from build123d import *

# Parameters (mm, degrees)
SKETCH_1_W      = 42
SKETCH_1_H      = 149
EXTRUDE_1_DEPTH = 3
SKETCH_2_W      = 25
SKETCH_2_H      = 12.5
EXTRUDE_2_DEPTH = 3
FILLET_1_R      = 1
SKETCH_3_W      = 6
SKETCH_3_H      = 4
EXTRUDE_3_DEPTH = 3
FILLET_2_R      = 2


with BuildPart() as part:
    # 草图1 → 凸台-拉伸1 (new body)
    with BuildSketch(Plane.XY):
        Rectangle(SKETCH_1_W, SKETCH_1_H)
    extrude(amount=EXTRUDE_1_DEPTH)

    # 草图2 → 凸台-拉伸2 (add)
    with BuildSketch(Plane.XY.offset(3)):
        with Locations((33.5, -68.25)):
            Rectangle(SKETCH_2_W, SKETCH_2_H)
        with Locations((-33.5, -68.25)):
            Rectangle(SKETCH_2_W, SKETCH_2_H)
        with Locations((-33.5, 68.25)):
            Rectangle(SKETCH_2_W, SKETCH_2_H)
        with Locations((33.5, 68.25)):
            Rectangle(SKETCH_2_W, SKETCH_2_H)
    extrude(amount=-EXTRUDE_2_DEPTH)

    # 圆角1
    fillet_1_edges = [part.edges().sort_by_distance(p)[0] for p in [
        (46, -74.5, 1.5),
        (46, -62, 1.5),
        (-46, -62, 1.5),
        (-46, -74.5, 1.5),
        (-46, 74.5, 1.5),
        (-46, 62, 1.5),
        (46, 62, 1.5),
        (46, 74.5, 1.5),
    ]]
    fillet(fillet_1_edges, radius=FILLET_1_R)

    # 草图3 → 凸台-拉伸3 (add)
    with BuildSketch(Plane(origin=(0, 0, 0), x_dir=(-1, 0, 0), z_dir=(0, 0, -1))):
        with Locations((38.15, 60)):
            Rectangle(SKETCH_3_W, SKETCH_3_H)
        with Locations((-38.15, 60)):
            Rectangle(SKETCH_3_W, SKETCH_3_H)
        with Locations((-38.15, -60)):
            Rectangle(SKETCH_3_W, SKETCH_3_H)
        with Locations((38.15, -60)):
            Rectangle(SKETCH_3_W, SKETCH_3_H)
    extrude(amount=-EXTRUDE_3_DEPTH)

    # 圆角2
    fillet_2_edges = [part.edges().sort_by_distance(p)[0] for p in [
        (-41.15, -58, 1.5),
        (-35.15, -58, 1.5),
        (-35.15, -62, 1.5),
        (41.15, -58, 1.5),
        (35.15, -62, 1.5),
        (35.15, -58, 1.5),
        (35.15, 58, 1.5),
        (41.15, 58, 1.5),
        (-35.15, 58, 1.5),
        (-35.15, 62, 1.5),
        (-41.15, 58, 1.5),
        (41.15, 62, 1.5),
    ]]
    fillet(fillet_2_edges, radius=FILLET_2_R - 0.0001)  # a hair under: the kernel refuses the full size


solid = part.part
Verification items for the finished model (mm, model axes). A direction names the side the tool comes from. Coordinates: 2 decimals unless noted, no trailing zeros. Order: outer loops, then holes, each group sorted by start corner. A loop starts at its lowest first (then second) coordinate and runs counter-clockwise, first axis right, second up. Notation, with made-up numbers: M 33,-39 L 46,-39 A24 cw 46,-8 Z; hole C 14,46.5 d3. An arc over 180 degrees is marked long. One line per item, written item: value. Start each with the question number.
Item 1: Depth check by flat-ended pin: P1, Ø1.5, axis at y = -12.5, z = 1.5, coming from the -X side; P2, Ø1, axis at y = -61, z = 1.5, coming from the -X side; P3, Ø0.6, axis at y = -61, z = 1, coming from the +X side. Enter the tip coordinate at first touch or a pass-through.
Item 2: Mould release check, pull along Y, two halves, no side actions. Record for faces 1 (the flat face through (-1, -74.5, 2)), 2 (the flat face through (21, -1, 1)), 3 (the flat face through (-46, 68, 2)): pulls with the +Y half, pulls with the -Y half, needs draft (parallel to the pull), parting line crosses it, or undercut.
Item 3: Thickness scan on probe 1 along Y at (x, z) = (27, 1.8); probe 2 along X at (y, z) = (23, 1.4); probe 3 along X at (y, z) = (59.5, 1.35). Record the ranges inside material, lowest first.
Item 4: Access from +Z, -Z, +X, -X, +Y, -Y to the whole of each face (thin tool, end or side, straight path). Record for faces 4 (the flat face through (-1, 1, 0)), 5 (the flat face through (28, 62, 2)), 6 (the flat face through (43, -62, 2)), 7 (the flat face through (-43, -62, 2)), 8 (the flat face through (-46, -68, 2)).
Item 5: Sectioned sample at A-A on y = -11.5. Record the cut outline in (x, z).
Calculated:
1. P1: x = -21
1. P2: x = -41.15
1. P3: x = 41.15
2. face 1: pulls with the -Y half
2. face 2: undercut
2. face 3: needs draft
3. probe 1: -74.5 to -62, 62 to 74.5
3. probe 2: -21 to 21
3. probe 3: -41.09 to -35.21, -21 to 21, 35.21 to 41.09
4. face 4: -Z, +X, -X, +Y, -Y
4. face 5: +Z, -Z
4. face 6: +Z, -Z, +X
4. face 7: +Z, -Z, -X
4. face 8: +Z, -Z, -X, +Y, -Y
5. outline: M -21,0 L 21,0 L 21,3 L -21,3 Z
